```python
from build123d import *

# Parameters (mm, degrees)
BOSS_EXTRUDE1_DEPTH = 1.5875
CUT_EXTRUDE2_DEPTH  = 109.601439476


with BuildPart() as part:
    # Sketch1 → Boss-Extrude1 (new body)
    with BuildSketch(Plane(origin=(0, 0, 0), x_dir=(1, 0, 0), z_dir=(0, 1, 0))):
        with BuildLine():
            Line((-35, -24.427940469), (-35, -71.7))
            ThreePointArc((-35, -71.7), (-34.414213562, -73.114213562), (-33, -73.7))
            Line((-33, -73.7), (-23, -73.7))
            ThreePointArc((-23, -73.7), (-21.585786438, -73.114213562), (-21, -71.7))
            Line((-21, -71.7), (-21, -30.7))
            ThreePointArc((-21, -30.7), (-20.414213562, -29.285786438), (-19, -28.7))
            Line((-19, -28.7), (19, -28.7))
            ThreePointArc((19, -28.7), (20.414213562, -29.285786438), (21, -30.7))
            Line((21, -30.7), (21, -71.7))
            ThreePointArc((21, -71.7), (21.585786438, -73.114213562), (23, -73.7))
            Line((23, -73.7), (33, -73.7))
            ThreePointArc((33, -73.7), (34.414213562, -73.114213562), (35, -71.7))
            Line((35, -71.7), (35, -24.427940469))
            ThreePointArc((35, -24.427940469), (35.120614758, -23.743900182), (35.467911114, -23.142365249))
            Line((35.467911114, -23.142365249), (42.282088886, -15.021544408))
            ThreePointArc((42.282088886, -15.021544408), (42.629385242, -14.420009476), (42.75, -13.735969189))
            Line((42.75, -13.735969189), (42.75, -2))
            ThreePointArc((42.75, -2), (42.164213562, -0.585786438), (40.75, 0))
            Line((40.75, 0), (-40.75, 0))
            ThreePointArc((-40.75, 0), (-42.164213562, -0.585786438), (-42.75, -2))
            Line((-42.75, -2), (-42.75, -13.735969189))
            ThreePointArc((-42.75, -13.735969189), (-42.629385242, -14.420009476), (-42.282088886, -15.021544408))
            Line((-42.282088886, -15.021544408), (-35.467911114, -23.142365249))
            ThreePointArc((-35.467911114, -23.142365249), (-35.120614758, -23.743900182), (-35, -24.427940469))
        make_face()
    extrude(amount=BOSS_EXTRUDE1_DEPTH)

    # Sketch3 → Cut-Extrude2 (cut, through all)
    with BuildSketch(Plane(origin=(37, 0, 0), x_dir=(0, 0, -1), z_dir=(1, 0, 0))):
        Polygon((-71.7, 1.5875), (-45.421699883, 1.5875), (-73.7, 0.6), (-73.7, 1.5875), align=None)
    extrude(amount=-CUT_EXTRUDE2_DEPTH, mode=Mode.SUBTRACT)


solid = part.part
```
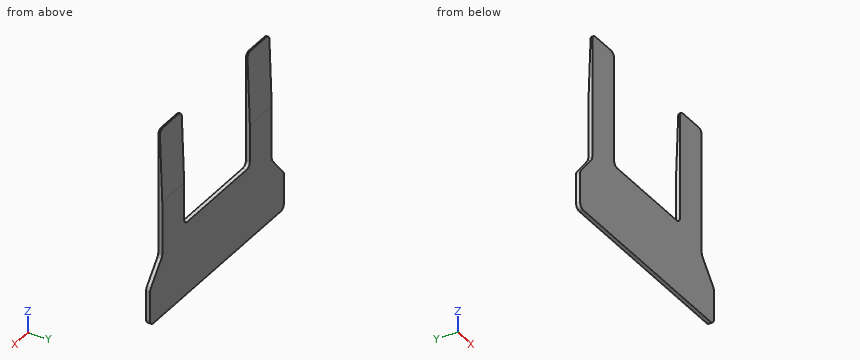
For this review, take the finished solid that the model builds, in its own axes (mm). Coordinates: 2 decimals unless noted, no trailing zeros. Write each loop counter-clockwise with the first axis right and the second up, starting at its lowest first coordinate (ties: lowest second). Pieces come first, ordered by that corner, then holes. Notation, with made-up numbers: (29, 77) - (54, 77) arc R28 ccw to (54, 112) - close; hole circle Ø10 at (79.5, 25). An arc over 180 degrees is marked (long way). Answer in a Markdown table with one row per item. Add a question column.
Q1. We need section C-C, the plane x = -26.5. State the section outline as (y, z) points, and give its area (3 significant figures).
Q2. For P1, Ø0.5, axis at x = 3.5, y = 1, coming from the +Z side; P2, Ø0.8, axis at y = 1, z = 54, coming from the +X side; P3, Ø0.5, axis at y = 0.5, z = 59, coming from the -X side; P4, Ø2, axis at x = 16.5, z = 14, coming from the -Y side, all flat-tipped, find the tip position at first contact; note any pin that passes through.
Q3. We need section B-B, the plane y = 0.3. State the section outline as (x, z) points, and give its area (3 significant figures).
Q4. We need section A-A, the plane z = 34.5. State the section outline as (x, y) points, and give its area (4 significant figures).
Q5. For probe 1 along X at (y, z) = (1.25, 32.5); probe 2 along Z at (x, y) = (2.5, 0.2); probe 3 along Y at (x, z) = (-33, 46), list the stretches that pass through material, from the lowest coordinate up.
Q6. We need section D-D, the plane z = 65. State the section outline as (x, y) points, and give its area (3 significant figures).
Answer list:
| question | item | result |
|---|---|---|
| 1 | outline | (0, 0) - (1.59, 0) - (1.59, 45.42) - (0.6, 73.7) - (0, 73.7) - close |
| 1 | area | 103 mm2 |
| 2 | P1 | stops at z = 28.7 |
| 2 | P2 | stops at x = 35 |
| 2 | P3 | stops at x = -35 |
| 2 | P4 | stops at y = 0 |
| 3 | outline | (-42.75, 2) arc R2 ccw to (-40.75, 0) - (40.75, 0) arc R2 ccw to (42.75, 2) - (42.75, 13.74) arc R2 ccw to (42.28, 15.02) - (35.47, 23.14) arc R2 cw to (35, 24.43) - (35, 71.7) arc R2 ccw to (33, 73.7) - (23, 73.7) arc R2 ccw to (21, 71.7) - (21, 30.7) arc R2 cw to (19, 28.7) - (-19, 28.7) arc R2 cw to (-21, 30.7) - (-21, 71.7) arc R2 ccw to (-23, 73.7) - (-33, 73.7) arc R2 ccw to (-35, 71.7) - (-35, 24.43) arc R2 cw to (-35.47, 23.14) - (-42.28, 15.02) arc R2 ccw to (-42.75, 13.74) - close |
| 3 | area | 3,560 mm2 |
| 4 | outline | (-35, 0) - (-21, 0) - (-21, 1.59) - (-35, 1.59) - close; (21, 0) - (35, 0) - (35, 1.59) - (21, 1.59) - close |
| 4 | area | 44.45 mm2 |
| 5 | probe 1 | x = -35 to -21, 21 to 35 |
| 5 | probe 2 | z = 0 to 28.7 |
| 5 | probe 3 | y = 0 to 1.57 |
| 6 | outline | (-35, 0) - (-21, 0) - (-21, 0.9) - (-35, 0.9) - close; (21, 0) - (35, 0) - (35, 0.9) - (21, 0.9) - close |
| 6 | area | 25.3 mm2 |
